Geometry check sheet. Reference: the model listing, model coordinates, mm. A direction names the side the tool comes from. Round coordinates to 2 decimals unless told otherwise and drop trailing zeros. Write each loop counter-clockwise with the first axis right and the second up, starting at its lowest first coordinate (ties: lowest second). Pieces come first, ordered by that corner, then holes. Notation, with made-up numbers: M 28,17.25 L 69,17.25 A14 cw 69,28.25 Z; hole C 42,74.5 d9. An arc over 180 degrees is marked long. Put each result on its own line as item: value. Start each with the question number.
(1) Gauge pin test, flat ends, axial feed: pin 1 (2.5 mm diameter, centred on x = 18, y = -116.5, fed in from +Z); pin 2 (3 mm diameter, centred on x = 20, y = -125, fed in from +Z); pin 3 (5 mm diameter, centred on x = 20, z = 37.5, fed in from +Y); pin 4 (5 mm diameter, centred on x = 21.5, z = 35.5, fed in from +Y). Record the tip position at first contact, or that the pin passes through.
(2) Section check D-D on y = -129. Record the cut outline in (x, z).
(3) Section check B-B on x = 19. Record the cut outline in (y, z) (3 decimals), then the cut area to 3 significant figures.
(4) Material ranges on probe 1 along X at (y, z) = (-88, 0.25); probe 2 along Z at (x, y) = (21, -139.65); probe 3 along X at (y, z) = (-139.15, 7.5), recorded low to high.
(5) Mould release check, pull along Z, two halves, no side actions. Record for faces 3 (the flat face through (21, -137, 7)), 4 (the flat face through (21, -137, 47)), 5 (the cylindrical face through (20.121, -85.253, -0.691)), 6 (the flat face through (20, -140, 60)): pulls with the +Z half, pulls with the -Z half, needs draft (parallel to the pull), parting line crosses it, or undercut.
(6) Section check A-A on y = -88. Record the cut outline in (x, z).
(7) Tool access check on faces 1 (the flat face through (25.5, -118, 21)), 2 (the flat face through (17, -120, 36)). Record the directions out of +Z, -Z, +X, -X, +Y, -Y that give a thin tool (end or side, any length) a straight path to the whole face; none if there is none.
(8) Section check C-C on z = 16. Record the cut outline in (x, y).
from build123d import *

# Parameters (mm, degrees)
SKETCH1_W           = 65
SKETCH1_H           = 57
BOSS_EXTRUDE1_DEPTH = 5
SKETCH2_W           = 65
SKETCH2_H           = 65
SKETCH2_R           = 2.75
SKETCH2_R_2         = 5
BOSS_EXTRUDE2_DEPTH = 5
SKETCH3_W           = 11
SKETCH3_H           = 60
BOSS_EXTRUDE7_DEPTH = 57
CUT_EXTRUDE2_DEPTH  = 165.705798319
SKETCH6_R           = 2.75
CUT_EXTRUDE3_DEPTH  = 89.911472826
SKETCH7_R           = 2.75
CUT_EXTRUDE4_DEPTH  = 160.515673211
CUT_EXTRUDE5_START  = 57
SKETCH8_W           = 11
SKETCH8_H           = 10
CUT_EXTRUDE5_DEPTH  = 40
CUT_EXTRUDE6_START  = 60
SKETCH9_W           = 11
SKETCH9_H           = 10
CUT_EXTRUDE6_DEPTH  = 56.5
SKETCH10_W          = 7
SKETCH10_H          = 62
SKETCH10_W_2        = 29
CUT_EXTRUDE7_DEPTH  = 160.515673211


with BuildPart() as part:
    # Sketch1 → Boss-Extrude1 (new body)
    with BuildSketch(Plane.XY):
        with Locations((0, -108.5)):
            Rectangle(SKETCH1_W, SKETCH1_H)
    extrude(amount=-BOSS_EXTRUDE1_DEPTH)

    # Sketch2 → Boss-Extrude2 (add)
    with BuildSketch(Plane.XZ.offset(137)):
        with Locations((0, 27.5)):
            Rectangle(SKETCH2_W, SKETCH2_H)
        with Locations(Location((20, 37.5, 0), (0, 0, 270))):
            Circle(SKETCH2_R, mode=Mode.SUBTRACT)
        with Locations(Location((21, 47.5, 0), (0, 0, 270))):
            Circle(SKETCH2_R_2, mode=Mode.SUBTRACT)
        with Locations(Location((-20, 47.5, 0), (0, 0, 270))):
            Circle(SKETCH2_R_2, mode=Mode.SUBTRACT)
        with Locations(Location((-20, 7.5, 0), (0, 0, 90))):
            Circle(SKETCH2_R_2, mode=Mode.SUBTRACT)
        with Locations(Location((21, 7.5, 0), (0, 0, 90))):
            Circle(SKETCH2_R_2, mode=Mode.SUBTRACT)
        with Locations(Location((-20, 37.5, 0), (0, 0, 90))):
            Circle(SKETCH2_R, mode=Mode.SUBTRACT)
    extrude(amount=BOSS_EXTRUDE2_DEPTH)

    # Sketch3 → Boss-Extrude7 (add)
    with BuildSketch(Plane(origin=(0, -137, 0), x_dir=(1, 0, 0), z_dir=(0, 1, 0))):
        with Locations((20, -30)):
            Rectangle(SKETCH3_W, SKETCH3_H)
        with Locations((-20, -30)):
            Rectangle(SKETCH3_W, SKETCH3_H)
    extrude(amount=BOSS_EXTRUDE7_DEPTH)

    # Sketch5 → Cut-Extrude2 (cut, through all)
    with BuildSketch(Plane(origin=(25.5, 0, 0), x_dir=(0, 0, -1), z_dir=(1, 0, 0))):
        Polygon((-60, -137), (0, -80), (-60, -80), align=None)
    extrude(amount=-CUT_EXTRUDE2_DEPTH, mode=Mode.SUBTRACT)

    # Sketch6 → Cut-Extrude3 (cut, through all)
    with BuildSketch(Plane.XZ.offset(137)):
        with Locations(Location((-20, 37.5, 0), (0, 0, 90))):
            Circle(SKETCH6_R)
        with Locations(Location((20, 37.5, 0), (0, 0, 90))):
            Circle(SKETCH6_R)
    extrude(amount=-CUT_EXTRUDE3_DEPTH, mode=Mode.SUBTRACT)

    # Sketch7 → Cut-Extrude4 (cut, through all)
    with BuildSketch(Plane.XY.offset(60)):
        with Locations((-20, -88)):
            Circle(SKETCH7_R)
        with Locations(Location((20, -88, 0), (0, 0, 270))):
            Circle(SKETCH7_R)
    extrude(amount=-CUT_EXTRUDE4_DEPTH, mode=Mode.SUBTRACT)

    # Sketch8 → Cut-Extrude5 (cut)
    with BuildSketch(Plane(origin=(0, -137, 0), x_dir=(1, 0, 0), z_dir=(0, 1, 0)).offset(CUT_EXTRUDE5_START)):
        with Locations((20, -37.5)):
            Rectangle(SKETCH8_W, SKETCH8_H)
        with Locations((-20, -37.5)):
            Rectangle(SKETCH8_W, SKETCH8_H)
    extrude(amount=-CUT_EXTRUDE5_DEPTH, mode=Mode.SUBTRACT)

    # Sketch9 → Cut-Extrude6 (cut)
    with BuildSketch(Plane.XY.offset(CUT_EXTRUDE6_START)):
        with Locations((-20, -88)):
            Rectangle(SKETCH9_W, SKETCH9_H)
        with Locations((20, -88)):
            Rectangle(SKETCH9_W, SKETCH9_H)
    extrude(amount=-CUT_EXTRUDE6_DEPTH, mode=Mode.SUBTRACT)

    # Sketch10 → Cut-Extrude7 (cut, through all)
    with BuildSketch(Plane.XY.offset(60)):
        with Locations((-29, -111)):
            Rectangle(SKETCH10_W, SKETCH10_H)
        with Locations((0, -111)):
            Rectangle(SKETCH10_W_2, SKETCH10_H)
        with Locations((29, -111)):
            Rectangle(SKETCH10_W, SKETCH10_H)
    extrude(amount=-CUT_EXTRUDE7_DEPTH, mode=Mode.SUBTRACT)


with BuildPart() as cut_extrude7_piece_1:
    # of the separate pieces the step leaves, piece 1, a body of its own (cut_extrude7_pieces)
    add(part.part.solids().sort_by_distance((25.5, -80, 0))[0])


with BuildPart() as cut_extrude7_piece_2:
    # of the separate pieces the step leaves, piece 2, a body of its own (cut_extrude7_pieces)
    add(part.part.solids().sort_by_distance((-14.5, -80, 0))[0])


solid = cut_extrude7_piece_1.part
Answers follow:
1. pin 1: stops at z = 32.5
1. pin 2: stops at z = 48.95
1. pin 3: passes through
1. pin 4: stops at y = -120
2. outline: M 14.5,-5 L 25.5,-5 L 25.5,51.58 L 14.5,51.58 Z; hole C 20,37.5 d5.5
3. outline: M -142,-5 L -90.562,-5 L -90.562,3.5 L -93,3.5 L -93,13.684 L -110.875,32.5 L -120,32.5 L -120,34.938 L -142,34.938 L -142,12.083 L -137,12.083 L -137,2.917 L -142,2.917 Z; M -142,40.062 L -120,40.062 L -120,42.105 L -137,60 L -142,60 L -142,52.083 L -137,52.083 L -137,42.917 L -142,42.917 Z; M -85.438,-5 L -80,-5 L -80,0 L -83.325,3.5 L -85.438,3.5 Z
3. area: 1,980 mm^2
4. probe 1: x = 14.5 to 17.25, 22.75 to 25.5
4. probe 2: z = -5 to 2.5, 12.5 to 34.94, 40.06 to 42.5, 52.5 to 60
4. probe 3: x = 14.5 to 16
5. face 3: undercut
5. face 4: undercut
5. face 5: needs draft
5. face 6: pulls with the +Z half
6. outline: M 14.5,-5 L 17.25,-5 L 17.25,3.5 L 14.5,3.5 Z; M 22.75,-5 L 25.5,-5 L 25.5,3.5 L 22.75,3.5 Z
7. face 1: +Z, -Z, +X, +Y, -Y
7. face 2: +Z, +X, -X, +Y
8. outline: M 14.5,-142 L 25.5,-142 L 25.5,-95.2 L 14.5,-95.2 Z
